CAD build for the part. Positions are in the model's coordinates, mm. A direction names the side the tool comes from. Give positions to 0.01 mm unless a question says otherwise; leave off trailing zeros. Order: outer loops, then holes, each group sorted by start corner. A loop starts at its lowest first (then second) coordinate and runs counter-clockwise, first axis right, second up.
Item 1: Band-saw the part on A-A on y = 28.1. Give the cut face in (x, z) (3 decimals).
Item 2: Band-saw the part on C-C on z = 1.75. Count the separate pieces of the cut face and the enclosed holes in it, plus the area to 3 significant figures.
Item 3: Wall check: L1, parallel to Y at x = 0, z = 2.5 (3 decimals); L2, parallel to X at y = -31, z = 1.65; L3, parallel to Y at x = 29.5, z = 1.75 (3 decimals). Give the ranges that are in metal, low to high.
Item 4: Which spindle directions (+Z, -Z, +X, -X, +Y, -Y) get a long thin tool onto all of the face, cutting with end or side? Do faces 1 (the cylindrical face through (-29.95, -23.55, 1.57)), 2 (the flat face through (0, -41.275, 2)). Say none if no direction does.
Item 5: Two-plate mould, pull along X, no slides. Class faces 3 (the flat face through (-0.5, 0.6, 3.175)), 4 (the flat face through (-35, -1, 2)), 5 (the cylindrical face through (3.23, 1.89, 1.57)): released by +X, released by -X, zero draft, split by the parting line, or undercut.
Item 6: Band-saw the part on B-B on x = 0. Give the cut face in (y, z) (3 decimals).
Item 7: Flat gauge pin, fed straight in: P1, Ø3, axis at x = 17.32, y = -1.9, coming from the -Z side. Where does the tip first touch, or does it go through?
Item 8: Band-saw the part on D-D on y = 8.1. Give the cut face in (x, z) (3 decimals), plus the area to 3 significant figures.
```python
from build123d import *

# Parameters (mm, degrees)
SKETCH1_W           = 70
SKETCH1_H           = 76.2
SKETCH1_R           = 1.75
SKETCH1_R_2         = 7
BOSS_EXTRUDE1_DEPTH = 3.175
SKETCH3_W           = 70
SKETCH3_H           = 3.175
BOSS_EXTRUDE2_DEPTH = 3.175


with BuildPart() as part:
    # Sketch1 → Boss-Extrude1 (new body)
    with BuildSketch(Plane.XY):
        Rectangle(SKETCH1_W, SKETCH1_H)
        with Locations((0, 28.1)):
            Circle(SKETCH1_R, mode=Mode.SUBTRACT)
        with Locations((17.320508076, -1.9)):
            Circle(SKETCH1_R, mode=Mode.SUBTRACT)
        with Locations((-17.320508076, -1.9)):
            Circle(SKETCH1_R, mode=Mode.SUBTRACT)
        with Locations((0, 8.1)):
            Circle(SKETCH1_R_2, mode=Mode.SUBTRACT)
        with BuildLine():
            Line((-32.05, 25.6), (-32.05, 30.6))
            ThreePointArc((-32.05, 30.6), (-30, 32.65), (-27.95, 30.6))
            Line((-27.95, 30.6), (-27.95, 25.6))
            ThreePointArc((-27.95, 25.6), (-30, 23.55), (-32.05, 25.6))
        make_face(mode=Mode.SUBTRACT)
        with BuildLine():
            Line((32.05, 25.6), (32.05, 30.6))
            ThreePointArc((32.05, 30.6), (30, 32.65), (27.95, 30.6))
            Line((27.95, 30.6), (27.95, 25.6))
            ThreePointArc((27.95, 25.6), (30, 23.55), (32.05, 25.6))
        make_face(mode=Mode.SUBTRACT)
        with BuildLine():
            Line((-32.05, -25.6), (-32.05, -30.6))
            ThreePointArc((-32.05, -30.6), (-30, -32.65), (-27.95, -30.6))
            Line((-27.95, -30.6), (-27.95, -25.6))
            ThreePointArc((-27.95, -25.6), (-30, -23.55), (-32.05, -25.6))
        make_face(mode=Mode.SUBTRACT)
        with BuildLine():
            Line((32.05, -25.6), (32.05, -30.6))
            ThreePointArc((32.05, -30.6), (30, -32.65), (27.95, -30.6))
            Line((27.95, -30.6), (27.95, -25.6))
            ThreePointArc((27.95, -25.6), (30, -23.55), (32.05, -25.6))
        make_face(mode=Mode.SUBTRACT)
    extrude(amount=BOSS_EXTRUDE1_DEPTH)

    # Sketch3 → Boss-Extrude2 (add)
    with BuildSketch(Plane.XY.offset(3.175)):
        with Locations((0, 39.6875)):
            Rectangle(SKETCH3_W, SKETCH3_H)
        with Locations((0, -39.6875)):
            Rectangle(SKETCH3_W, SKETCH3_H)
    extrude(amount=-BOSS_EXTRUDE2_DEPTH)


solid = part.part
```
The answers:
1. outline: (-35, 0) - (-32.05, 0) - (-32.05, 3.175) - (-35, 3.175) - close; (-27.95, 0) - (-1.75, 0) - (-1.75, 3.175) - (-27.95, 3.175) - close; (1.75, 0) - (27.95, 0) - (27.95, 3.175) - (1.75, 3.175) - close; (32.05, 0) - (35, 0) - (35, 3.175) - (32.05, 3.175) - close
2. separate pieces: 1
2. enclosed holes: 8
2. area: 5,460 mm2
3. L1: y = -41.275 to 1.1, 15.1 to 26.35, 29.85 to 41.275
3. L2: x = -35 to -32.01, -27.99 to 27.99, 32.01 to 35
3. L3: y = -41.275 to -32.588, -23.612 to 23.612, 32.588 to 41.275
4. face 1: +Z, -Z
4. face 2: +Z, -Z, +X, -X, -Y
5. face 3: zero draft
5. face 4: released by -X
5. face 5: undercut
6. outline: (-41.275, 0) - (1.1, 0) - (1.1, 3.175) - (-41.275, 3.175) - close; (15.1, 0) - (26.35, 0) - (26.35, 3.175) - (15.1, 3.175) - close; (29.85, 0) - (41.275, 0) - (41.275, 3.175) - (29.85, 3.175) - close
7. P1: passes through
8. outline: (-35, 0) - (-7, 0) - (-7, 3.175) - (-35, 3.175) - close; (7, 0) - (35, 0) - (35, 3.175) - (7, 3.175) - close
8. area: 178 mm2
